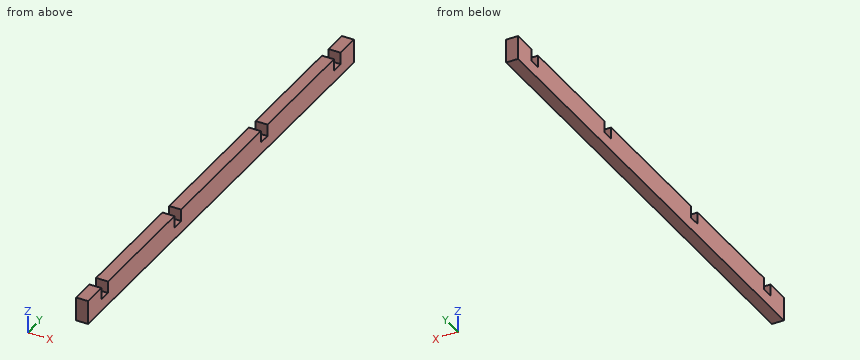
from build123d import *

# Parameters (mm, degrees)
F0_W     = 1016
F0_H     = 50.8
F1_DEPTH = 25.4
F2_W     = 25.4
F2_H     = 25.4
F3_DEPTH = 25.4
F4_W     = 25.4
F4_H     = 25.4
F5_DEPTH = 25.4


with BuildPart() as f1:
    # F0 (on Right) → F1 (new body)
    with BuildSketch(Plane.YZ):
        Rectangle(F0_W, F0_H)
    extrude(amount=F1_DEPTH)

    # F2 (on face) → F3 (cut)
    with BuildSketch(Plane.YZ.offset(25.4)):
        with Locations((-165.1, 12.7)):
            Rectangle(F2_W, F2_H)
        with Locations((165.1, 12.7)):
            Rectangle(F2_W, F2_H)
    extrude(amount=-F3_DEPTH, mode=Mode.SUBTRACT)

    # F4 (on face) → F5 (cut)
    with BuildSketch(Plane.YZ.offset(25.4)):
        with Locations((-444.5, 12.7)):
            Rectangle(F4_W, F4_H)
        with Locations((444.5, 12.7)):
            Rectangle(F4_W, F4_H)
    extrude(amount=-F5_DEPTH, mode=Mode.SUBTRACT)


solid = f1.part
CAD build for the part. Positions are in the model's coordinates, mm. Give positions to 0.01 mm unless a question says otherwise; leave off trailing zeros. Loops run counter-clockwise (first coordinate to the right, second up) from the corner with the lowest first, then second, coordinate; pieces in that order, holes last. Notation, with made-up numbers: M -28,-39 L -8,-39 A12 ccw -8,-17 Z; hole C 9.25,-11.75 d2. An arc over 180 degrees is marked long. One line per question, with ' | ' between items. Start each with the question number.
1. Flat gauge pin, fed straight in: pin 1 (7.5 mm diameter, centred on x = 14, y = -159.5, fed in from +Z). Where does the tip first touch, or does it go through?
2. Probe L1, parallel to Y at x = 13.75, z = 21; L2, parallel to Z at x = 19.25, y = 443. List the from-to ranges inside material, lowest first. Write a range as from..to.
3. Saw through at B-B on x = 20. Give the cut face in (y, z).
4. Saw through at A-A on z = 13. Give the cut face in (x, y), plus the area to 3 significant figures.
Result sheet:
1) pin 1: stops at z = 0
2) L1: y = -508..-457.2, -431.8..-177.8, -152.4..152.4, 177.8..431.8, 457.2..508 | L2: z = -25.4..0
3) outline: M -508,-25.4 L 508,-25.4 L 508,25.4 L 457.2,25.4 L 457.2,0 L 431.8,0 L 431.8,25.4 L 177.8,25.4 L 177.8,0 L 152.4,0 L 152.4,25.4 L -152.4,25.4 L -152.4,0 L -177.8,0 L -177.8,25.4 L -431.8,25.4 L -431.8,0 L -457.2,0 L -457.2,25.4 L -508,25.4 Z
4) outline: M 0,-508 L 25.4,-508 L 25.4,-457.2 L 0,-457.2 Z; M 0,-431.8 L 25.4,-431.8 L 25.4,-177.8 L 0,-177.8 Z; M 0,-152.4 L 25.4,-152.4 L 25.4,152.4 L 0,152.4 Z; M 0,177.8 L 25.4,177.8 L 25.4,431.8 L 0,431.8 Z; M 0,457.2 L 25.4,457.2 L 25.4,508 L 0,508 Z | area: 23,200 mm^2
